from build123d import *

# Parameters (mm, degrees)
ESQUISSE1_R        = 1.1
BOSS_EXTRU_1_DEPTH = 0.8


with BuildPart() as part:
    # Esquisse1 → Boss.-Extru.1 (new body, symmetric)
    with BuildSketch(Plane(origin=(0, 0, 0), x_dir=(1, 0, 0), z_dir=(0, 1, 0))):
        with BuildLine():
            ThreePointArc((-2, -10), (0, -12), (2, -10))
            Line((2, -10), (9.2, -10))
            ThreePointArc((9.2, -10), (9.765685425, -9.765685425), (10, -9.2))
            Line((10, -9.2), (10, -2.1))
            ThreePointArc((10, -2.1), (7.9, 0), (10, 2.1))
            Line((10, 2.1), (10, 9.2))
            ThreePointArc((10, 9.2), (9.765685425, 9.765685425), (9.2, 10))
            Line((9.2, 10), (2, 10))
            ThreePointArc((2, 10), (0, 12), (-2, 10))
            Line((-2, 10), (-9.2, 10))
            ThreePointArc((-9.2, 10), (-9.765685425, 9.765685425), (-10, 9.2))
            Line((-10, 9.2), (-10, 2.1))
            ThreePointArc((-10, 2.1), (-7.9, 0), (-10, -2.1))
            Line((-10, -2.1), (-10, -9.2))
            ThreePointArc((-10, -9.2), (-9.765685425, -9.765685425), (-9.2, -10))
            Line((-9.2, -10), (-2, -10))
        make_face()
        with Locations((0, -10)):
            Circle(ESQUISSE1_R, mode=Mode.SUBTRACT)
        with Locations((0, 10)):
            Circle(ESQUISSE1_R, mode=Mode.SUBTRACT)
    extrude(amount=BOSS_EXTRU_1_DEPTH, both=True)


solid = part.part
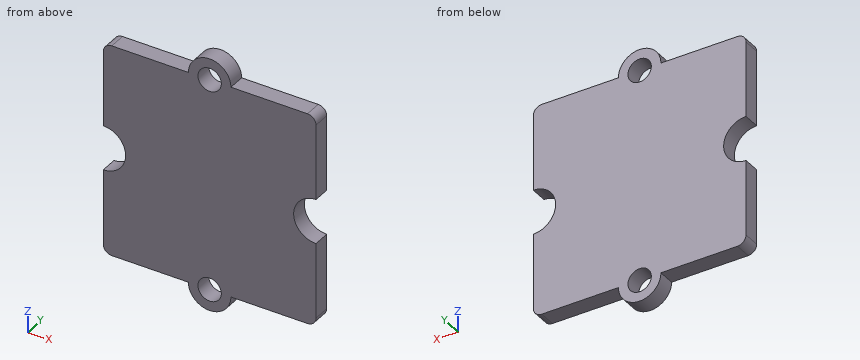
Design review of the part built by this model. Coordinates are the model's own, in mm. Give positions to 0.01 mm unless a question says otherwise; leave off trailing zeros. Loops run counter-clockwise (first coordinate to the right, second up) from the corner with the lowest first, then second, coordinate; pieces in that order, holes last. Notation, with made-up numbers: (-34.75, 4) - (24.25, 4) arc R20 ccw to (24.25, 15) - close; hole circle Ø4 at (-8.75, 61.5). An arc over 180 degrees is marked (long way). Use CSV: the item, a comma, the result in double quotes. Start each with the question number.
1. Wall thickness on L1, parallel to Z at x = 0, y = -0.4; L2, parallel to Z at x = 2.25, y = -0.5; L3, parallel to Z at x = -0.5, y = -0.4: over which ranges is each line inside the solid? List them lowest first.
2. Add section A-A (y = 0). State the section outline as (x, z) points.
3. Insertion check: P1, Ø0.5, axis at x = -6, y = 0, coming from the +Z side; P2, Ø3, axis at x = 0, z = 10, coming from the -Y side; P3, Ø0.5, axis at x = 6.5, y = 0, coming from the -Z side. Each pin has a flat end and moves straight along its axis. Give the tip position at first contact, or say it passes through.
4. Add section D-D (z = 0). State the section outline as (x, y) points.
5. Add section C-C (x = -3.5). State the section outline as (y, z) points.
6. Add section B-B (z = 10.75). State the section outline as (x, y) points.
Results found:
1,L1,"z = -12 to -11.1, -8.9 to 8.9, 11.1 to 12"
1,L2,"z = -10 to 10"
1,L3,"z = -11.94 to -10.98, -9.02 to 9.02, 10.98 to 11.94"
2,outline,"(-10, -9.2) arc R0.8 ccw to (-9.2, -10) - (-2, -10) arc R2 ccw to (2, -10) - (9.2, -10) arc R0.8 ccw to (10, -9.2) - (10, -2.1) arc R2.1 cw to (10, 2.1) - (10, 9.2) arc R0.8 ccw to (9.2, 10) - (2, 10) arc R2 ccw to (-2, 10) - (-9.2, 10) arc R0.8 ccw to (-10, 9.2) - (-10, 2.1) arc R2.1 cw to (-10, -2.1) - close; hole circle Ø2.2 at (0, -10); hole circle Ø2.2 at (0, 10)"
3,P1,"stops at z = 10"
3,P2,"stops at y = -0.8"
3,P3,"stops at z = -10"
4,outline,"(-7.9, -0.8) - (7.9, -0.8) - (7.9, 0.8) - (-7.9, 0.8) - close"
5,outline,"(-0.8, -10) - (0.8, -10) - (0.8, 10) - (-0.8, 10) - close"
6,outline,"(-1.85, -0.8) - (-0.8, -0.8) - (-0.8, 0.8) - (-1.85, 0.8) - close; (0.8, -0.8) - (1.85, -0.8) - (1.85, 0.8) - (0.8, 0.8) - close"
